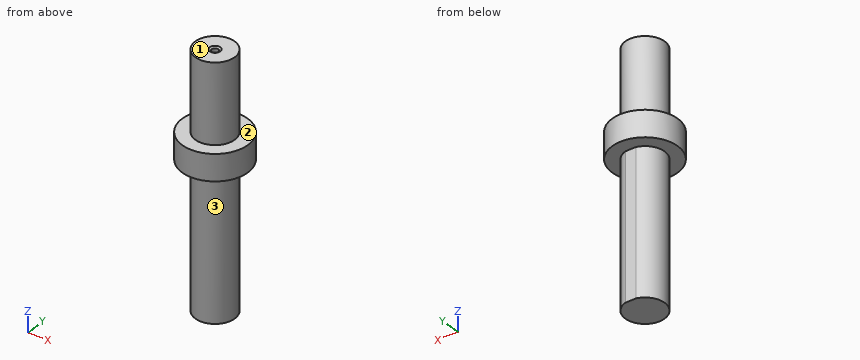
from build123d import *

# Parameters (mm, degrees)
SKETCH1_R                       = 12.5
F_25MM_DIA_DEPTH                = 10
F_15MM_START                    = -10
SKETCH2_R                       = 7.5
F_15MM_DIA_BEARING_END_DEPTH    = 40
F_15MM_START_2                  = 55
SKETCH3_R                       = 7.5
F_15MM_DIA_GEAR_END_DEPTH       = 55
M3X0_5_TAPPED_HOLE1_D           = 2.5
M3X0_5_TAPPED_HOLE1_DEPTH       = 15
M3X0_5_TAPPED_HOLE1_CSINK_D     = 4
M3X0_5_TAPPED_HOLE1_CSINK_ANGLE = 120
M3X0_5_TAPPED_HOLE1_TIP         = 0.751075774
SKETCH8_W                       = 4
SKETCH8_H                       = 3.025433208
CUT_EXTRUDE1_DEPTH              = 55


with BuildPart() as part:
    # Sketch1 → 25mm dia (new body)
    with BuildSketch(Plane.XY):
        Circle(SKETCH1_R)
    extrude(amount=F_25MM_DIA_DEPTH)

    # Sketch2 → 15mm dia bearing end (add)
    with BuildSketch(Plane.XY.offset(10).offset(F_15MM_START)):
        Circle(SKETCH2_R)
    extrude(amount=F_15MM_DIA_BEARING_END_DEPTH)

    # Sketch3 → 15mm dia gear end (add)
    with BuildSketch(Plane(origin=(0, 0, 0), x_dir=(-1, 0, 0), z_dir=(0, 0, -1)).offset(F_15MM_START_2)):
        with Locations(Location((0, 0, 0), (0, 0, 180))):
            Circle(SKETCH3_R)
    extrude(amount=-F_15MM_DIA_GEAR_END_DEPTH)

    # M3x0.5 Tapped Hole1
    with Locations(Plane.XY.offset(40)):
        with Locations((0, 0)):
            CounterSinkHole(M3X0_5_TAPPED_HOLE1_D / 2, M3X0_5_TAPPED_HOLE1_CSINK_D / 2, depth=M3X0_5_TAPPED_HOLE1_DEPTH, counter_sink_angle=M3X0_5_TAPPED_HOLE1_CSINK_ANGLE)
            with Locations((0, 0, -(M3X0_5_TAPPED_HOLE1_DEPTH + M3X0_5_TAPPED_HOLE1_TIP / 2))):  # 118° drill point
                Cone(0, M3X0_5_TAPPED_HOLE1_D / 2, M3X0_5_TAPPED_HOLE1_TIP, mode=Mode.SUBTRACT)

    # Sketch8 → Cut-Extrude1 (cut)
    with BuildSketch(Plane(origin=(0, 0, -55), x_dir=(-1, 0, 0), z_dir=(0, 0, -1))):
        with Locations((0, 8.741132751)):
            Rectangle(SKETCH8_W, SKETCH8_H)
    extrude(amount=-CUT_EXTRUDE1_DEPTH, mode=Mode.SUBTRACT)


solid = part.part
Could you check a few things on this model? Use its own coordinates, in mm. Face numbers are marked on the shaded views. A direction names the side the tool comes from. Give positions to 0.01 mm unless a question says otherwise; leave off trailing zeros. Order: outer loops, then holes, each group sorted by start corner. A loop starts at its lowest first (then second) coordinate and runs counter-clockwise, first axis right, second up. Notation, with made-up numbers: (75, 15) -> (122, 15) arc R12 ccw to (122, 32) -> close; hole circle Ø4 at (43.5, 68). An arc over 180 degrees is marked (long way). Return JSON: item names as keys, results as strings.
1. On a 3-axis mill with a long thin cutter (end or side, diameter ignored), from which of +Z, -Z, +X, -X, +Y, -Y can I reach the whole of each face in a straight line? I mean the marked faces 1, 2 and 3. Say none if no direction works.
Answer list:
{"face 1": "+Z, +X, -X, +Y, -Y", "face 2": "+Z", "face 3": "-Z"}
2. For pin 1 Ø2 at (x, z) = (5.5, 3) entering from -Y; pin 2 Ø2 at (x, z) = (0.5, -38) entering from +Y; pin 3 Ø2 at (x, y) = (5, 9.5) entering from -Z, each with a flat end and sliding along its axis, tell me the tip position at first contact or that it passes through.
Answer list:
{"pin 1": "stops at y = -11.66", "pin 2": "stops at y = 7.23", "pin 3": "stops at z = 0"}
3. Imagine slicing it at B-B on x = 6.25. List the corners of the cut face in (y, z) for me.
Answer list:
{"outline": "(-10.83, 0) -> (-4.15, 0) -> (-4.15, -55) -> (4.15, -55) -> (4.15, 0) -> (10.83, 0) -> (10.83, 10) -> (4.15, 10) -> (4.15, 40) -> (-4.15, 40) -> (-4.15, 10) -> (-10.83, 10) -> close"}
4. Imagine slicing it at D-D on z = -12. List the corners of the cut face in (x, y) for me.
Answer list:
{"outline": "(-2, 7.23) arc R7.5 ccw (long way) to (2, 7.23) -> close"}
5. I need wall thicknesses on line 1 (X direction, y = 0, z = 29.5); line 2 (X direction, y = -0.25, z = -25.5). Which ranges of each line are inside material? Lowest first, please. Write a range as from..to.
Answer list:
{"line 1": "x = -7.5..-1.25, 1.25..7.5", "line 2": "x = -7.5..7.5"}
6. Imagine slicing it at C-C on z = 14. List the corners of the cut face in (x, y) for me.
Answer list:
{"outline": "circle Ø15 at (0, 0)"}
7. Imagine slicing it at A-A on y = -5.5. List the corners of the cut face in (x, z) for me.
Answer list:
{"outline": "(-11.22, 0) -> (-5.1, 0) -> (-5.1, -55) -> (5.1, -55) -> (5.1, 0) -> (11.22, 0) -> (11.22, 10) -> (5.1, 10) -> (5.1, 40) -> (-5.1, 40) -> (-5.1, 10) -> (-11.22, 10) -> close"}
